Geometry check sheet. Reference: the model listing, model coordinates, mm. A direction names the side the tool comes from. Give positions to 0.01 mm unless a question says otherwise; leave off trailing zeros. Loops run counter-clockwise (first coordinate to the right, second up) from the corner with the lowest first, then second, coordinate; pieces in that order, holes last. Notation, with made-up numbers: (-4, 70.5) -> (41, 70.5) arc R24 ccw to (41, 88.5) -> close; hole circle Ø11 at (-22.5, 6). An arc over 180 degrees is marked (long way). Write each question's results on one line, items separated by ' | '. Start each with the question number.
1) Depth check by flat-ended pin: pin 1 (3 mm diameter, centred on y = -7, z = -14.5, fed in from +X); pin 2 (10 mm diameter, centred on x = -9, y = -4, fed in from -Z); pin 3 (4 mm diameter, centred on y = -15.5, z = -6.5, fed in from -X). Enter the tip coordinate at first touch or a pass-through.
2) Sectioned sample at B-B on x = 0. Record the cut outline in (y, z), then the cut area to 4 significant figures.
3) Scan lines: line 1 (Y direction, x = 14, z = -18.5); line 2 (X direction, y = 0, z = 4); line 3 (Z direction, x = 13, y = -23). Record each from-to range of solid material in increasing order. Write a range as from..to.
4) Sectioned sample at C-C on y = -2.5. Record the cut outline in (x, z).
5) Sectioned sample at A-A on z = 0. Record the cut outline in (x, y), then the cut area to 4 significant figures.
6) Set-up check for faces 1 (the face through (0, -25, 0)), 2 (the face through (-4.769, -19.93, -21.477)): record each of +Z, -Z, +X, -X, +Y, -Y from which the full face is reachable in a straight line by a thin tool's end or side.
```python
from build123d import *

# Parameters (mm, degrees)
F0_R     = 22
F2_DEPTH = 25
F3_DEPTH = 25
F4_R     = 24.5
F5_DEPTH = 25


with BuildPart() as f2:
    # F0 (on Front) → F2 (new body)
    with BuildSketch(Plane.XZ):
        Circle(F0_R)
        with BuildLine():
            ThreePointArc((-19.401899791, 1.9535312895), (-13.921825835, 13.654038429), (-2.3299484959, 19.3603032003))
            ThreePointArc((-2.3299484959, 19.3603032003), (0, 19.5), (2.3299484959, 19.3603032003))
            ThreePointArc((2.3299484959, 19.3603032003), (13.921825835, 13.654038429), (19.401899791, 1.9535312895))
            ThreePointArc((19.401899791, 1.9535312895), (19.4754595058, 0.9779964404), (19.5, 0))
            ThreePointArc((19.5, 0), (19.4754595058, -0.9779964404), (19.401899791, -1.9535312895))
            ThreePointArc((19.401899791, -1.9535312895), (13.921825835, -13.654038429), (2.3299484959, -19.3603032003))
            ThreePointArc((2.3299484959, -19.3603032003), (0, -19.5), (-2.3299484959, -19.3603032003))
            ThreePointArc((-2.3299484959, -19.3603032003), (-13.921825835, -13.654038429), (-19.401899791, -1.9535312895))
            ThreePointArc((-19.401899791, -1.9535312895), (-19.5, 0), (-19.401899791, 1.9535312895))
        make_face(mode=Mode.SUBTRACT)
    extrude(amount=F2_DEPTH)



with BuildPart() as f2b:
    # F0 (on Front) → F2, piece 2 (new body)
    with BuildSketch(Plane.XZ):
        with BuildLine():
            ThreePointArc((-2.8938206378, 1.9535312895), (-1.7519205381, 1.9616594322), (-1.1833040417, 2.9519508966))
            ThreePointArc((-1.1833040417, 2.9519508966), (-1.5191484267, 3.7627509657), (-2.3299484959, 4.0985953507))
            ThreePointArc((-2.3299484959, 4.0985953507), (-3.4389177943, 3.2434652177), (-2.8938206378, 1.9535312895))
        make_face()
    extrude(amount=F2_DEPTH)


with BuildPart() as f2_1:
    add(f2.part)

    add(f2b.part)  # F3 merges F2b
    # F0 (on Front) → F3 (join)
    with BuildSketch(Plane.XZ):
        with BuildLine():
            ThreePointArc((-2.8938206378, 1.9535312895), (-3.4389177943, 3.2434652177), (-2.3299484959, 4.0985953507))
            Line((-2.3299484959, 4.0985953507), (-2.3299484959, 19.3603032003))
            ThreePointArc((-2.3299484959, 19.3603032003), (-13.921825835, 13.654038429), (-19.401899791, 1.9535312895))
            Line((-19.401899791, 1.9535312895), (-2.8938206378, 1.9535312895))
        make_face()
        with BuildLine():
            ThreePointArc((19.401899791, 1.9535312895), (13.921825835, 13.654038429), (2.3299484959, 19.3603032003))
            Line((2.3299484959, 19.3603032003), (2.3299484959, 4.0985953507))
            ThreePointArc((2.3299484959, 4.0985953507), (3.140748565, 3.7627509657), (3.47659295, 2.9519508966))
            ThreePointArc((3.47659295, 2.9519508966), (3.3202399602, 2.3739229388), (2.8938206378, 1.9535312895))
            Line((2.8938206378, 1.9535312895), (19.401899791, 1.9535312895))
        make_face()
        with BuildLine():
            ThreePointArc((-2.3299484959, 4.0985953507), (-1.5191484267, 3.7627509657), (-1.1833040417, 2.9519508966))
            ThreePointArc((-1.1833040417, 2.9519508966), (-1.7519205381, 1.9616594322), (-2.8938206378, 1.9535312895))
            Line((-2.8938206378, 1.9535312895), (-19.401899791, 1.9535312895))
            ThreePointArc((-19.401899791, 1.9535312895), (-19.5, 0), (-19.401899791, -1.9535312895))
            Line((-19.401899791, -1.9535312895), (-2.8938206378, -1.9535312895))
            ThreePointArc((-2.8938206378, -1.9535312895), (-1.7519205381, -1.9616594322), (-1.1833040417, -2.9519508966))
            ThreePointArc((-1.1833040417, -2.9519508966), (-1.5191484267, -3.7627509657), (-2.3299484959, -4.0985953507))
            Line((-2.3299484959, -4.0985953507), (-2.3299484959, -19.3603032003))
            ThreePointArc((-2.3299484959, -19.3603032003), (0, -19.5), (2.3299484959, -19.3603032003))
            Line((2.3299484959, -19.3603032003), (2.3299484959, -4.0985953507))
            ThreePointArc((2.3299484959, -4.0985953507), (1.2209791974, -2.6604365754), (2.8938206378, -1.9535312895))
            Line((2.8938206378, -1.9535312895), (19.401899791, -1.9535312895))
            ThreePointArc((19.401899791, -1.9535312895), (19.4754595058, -0.9779964404), (19.5, 0))
            ThreePointArc((19.5, 0), (19.4754595058, 0.9779964404), (19.401899791, 1.9535312895))
            Line((19.401899791, 1.9535312895), (2.8938206378, 1.9535312895))
            ThreePointArc((2.8938206378, 1.9535312895), (1.2209791974, 2.6604365754), (2.3299484959, 4.0985953507))
            Line((2.3299484959, 4.0985953507), (2.3299484959, 19.3603032003))
            ThreePointArc((2.3299484959, 19.3603032003), (0, 19.5), (-2.3299484959, 19.3603032003))
            Line((-2.3299484959, 19.3603032003), (-2.3299484959, 4.0985953507))
        make_face()
        with BuildLine():
            Line((-2.8938206378, -1.9535312895), (-19.401899791, -1.9535312895))
            ThreePointArc((-19.401899791, -1.9535312895), (-13.921825835, -13.654038429), (-2.3299484959, -19.3603032003))
            Line((-2.3299484959, -19.3603032003), (-2.3299484959, -4.0985953507))
            ThreePointArc((-2.3299484959, -4.0985953507), (-3.4389177943, -3.2434652177), (-2.8938206378, -1.9535312895))
        make_face()
        with BuildLine():
            Line((2.3299484959, -4.0985953507), (2.3299484959, -19.3603032003))
            ThreePointArc((2.3299484959, -19.3603032003), (13.921825835, -13.654038429), (19.401899791, -1.9535312895))
            Line((19.401899791, -1.9535312895), (2.8938206378, -1.9535312895))
            ThreePointArc((2.8938206378, -1.9535312895), (3.3202399602, -2.3739229388), (3.47659295, -2.9519508966))
            ThreePointArc((3.47659295, -2.9519508966), (3.140748565, -3.7627509657), (2.3299484959, -4.0985953507))
        make_face()
        with BuildLine():
            ThreePointArc((2.8938206378, -1.9535312895), (1.2209791974, -2.6604365754), (2.3299484959, -4.0985953507))
            ThreePointArc((2.3299484959, -4.0985953507), (3.140748565, -3.7627509657), (3.47659295, -2.9519508966))
            ThreePointArc((3.47659295, -2.9519508966), (3.3202399602, -2.3739229388), (2.8938206378, -1.9535312895))
        make_face()
        with BuildLine():
            ThreePointArc((3.47659295, 2.9519508966), (3.140748565, 3.7627509657), (2.3299484959, 4.0985953507))
            ThreePointArc((2.3299484959, 4.0985953507), (1.2209791974, 2.6604365754), (2.8938206378, 1.9535312895))
            ThreePointArc((2.8938206378, 1.9535312895), (3.3202399602, 2.3739229388), (3.47659295, 2.9519508966))
        make_face()
        with BuildLine():
            ThreePointArc((-1.1833040417, -2.9519508966), (-1.7519205381, -1.9616594322), (-2.8938206378, -1.9535312895))
            ThreePointArc((-2.8938206378, -1.9535312895), (-3.4389177943, -3.2434652177), (-2.3299484959, -4.0985953507))
            ThreePointArc((-2.3299484959, -4.0985953507), (-1.5191484267, -3.7627509657), (-1.1833040417, -2.9519508966))
        make_face()
    extrude(amount=F3_DEPTH)

    # F4 (on offset) → F5 (join)
    with BuildSketch(Plane.XZ.offset(15)):
        Circle(F4_R)
    extrude(amount=-F5_DEPTH)


solid = f2_1.part
```
Result:
1) pin 1: x = 20.77 | pin 2: z = -24.17 | pin 3: x = -24.07
2) outline: (-25, -22) -> (-15, -22) -> (-15, -24.5) -> (10, -24.5) -> (10, 24.5) -> (-15, 24.5) -> (-15, 22) -> (-25, 22) -> close | area: 1,665 mm^2
3) line 1: -15..10 | line 2: -24.17..24.17 | line 3: -17.75..17.75
4) outline: circle Ø49 at (0, 0)
5) outline: (-24.5, -15) -> (-22, -15) -> (-22, -25) -> (22, -25) -> (22, -15) -> (24.5, -15) -> (24.5, 10) -> (-24.5, 10) -> close | area: 1,665 mm^2
6) face 1: +Z, -Z, +X, -X, -Y | face 2: -Y
